```python
from build123d import *

# Parameters (mm, degrees)
F0_R     = 14.097
F0_R_2   = 14.1605
F0_R_3   = 14.224
F0_R_4   = 14.2875
F0_W     = 6.604
F0_H     = 13.208
F0_R_5   = 14.351
F0_H_2   = 12.954
F0_R_6   = 14.4145
F0_R_7   = 14.478
F1_DEPTH = 6.604


with BuildPart() as f1:
    # F0 (on Top) → F1 (new body)
    with BuildSketch(Plane.XY):
        with BuildLine():
            ThreePointArc((25.4, 123.19), (24.284077, 125.884077), (21.59, 127))
            Line((21.59, 127), (6.239323, 127))
            Line((6.239323, 127), (6.239323, 133.604))
            Line((6.239323, 133.604), (-6.460677, 133.604))
            Line((-6.460677, 133.604), (-6.460677, 127))
            Line((-6.460677, 127), (-21.59, 127))
            ThreePointArc((-21.59, 127), (-24.284077, 125.884077), (-25.4, 123.19))
            Line((-25.4, 123.19), (-25.4, -123.19))
            ThreePointArc((-25.4, -123.19), (-24.284077, -125.884077), (-21.59, -127))
            Line((-21.59, -127), (21.59, -127))
            ThreePointArc((21.59, -127), (24.284077, -125.884077), (25.4, -123.19))
            Line((25.4, -123.19), (25.4, 123.19))
        make_face()
        with Locations((0, -105.552882)):
            Circle(F0_R, mode=Mode.SUBTRACT)
        with Locations((0, -72.061613)):
            Circle(F0_R_2, mode=Mode.SUBTRACT)
        with Locations((0, -37.917089)):
            Circle(F0_R_3, mode=Mode.SUBTRACT)
        Circle(F0_R_4, mode=Mode.SUBTRACT)
        with Locations((20.013824, -19.935825)):
            Rectangle(F0_W, F0_H, mode=Mode.SUBTRACT)
        with Locations((0, 36.432702)):
            Circle(F0_R_5, mode=Mode.SUBTRACT)
        with Locations((18.755223, 17.765409)):
            Rectangle(F0_W, F0_H_2, mode=Mode.SUBTRACT)
        with Locations((0, 71.722105)):
            Circle(F0_R_6, mode=Mode.SUBTRACT)
        with Locations((0, 107.080773)):
            Circle(F0_R_7, mode=Mode.SUBTRACT)
    extrude(amount=F1_DEPTH)


solid = f1.part
```
Could you check a few things on this model? Use its own coordinates, in mm. A direction names the side the tool comes from. Coordinates: 2 decimals unless noted, no trailing zeros. Order: outer loops, then holes, each group sorted by start corner. A loop starts at its lowest first (then second) coordinate and runs counter-clockwise, first axis right, second up. Notation, with made-up numbers: M -22.5,65 L -17.5,65 A32 cw -17.5,100 Z; hole C 8,-19 d6. An arc over 180 degrees is marked long. Use a Markdown table: item, result. Add a question column.
Q1. We'd pull the mould along X, two halves only. Please class faces 5 (the flat face through (-17, 5, 6.604)), 6 (the cylindrical face through (-3.139, 92.947, 3.256)), 7 (the flat face through (6.239, 130, 3)): pulls with the +X half, pulls with the -X half, needs draft (parallel to the pull), parting line crosses it, or undercut.
Q2. I want a section at B-B on y = 0. List the corners of the cut face in (x, z) for me, then the cut area to 3 significant figures.
Q3. If I drill on L1, parallel to Y at x = 21, z = 1.25; L2, parallel to X at y = 105, z = 3.5; L3, parallel to Y at x = 16, z = 0.5, over which ranges is the centre line in solid material (lowest first)?
Q4. I want a section at A-A on x = 0. Give the number of separate pieces and of enclosed holes in the cut face, then the cut area to 3 significant figures.
Q5. I'm going to push flat-ended pins straight in: pin 1 (3.5 mm diameter, centred on x = -11, z = 3, fed in from +Y); pin 2 (6 mm diameter, centred on x = -13, y = -80, fed in from -Z). Where does each tip first touch, or does it pass through?
Q6. I want a section at D-D on y = 103. List the corners of the cut face in (x, z) for me, then the cut area to 3 significant figures.
Q7. Which directions (+Z, -Z, +X, -X, +Y, -Y) give clear straight access to the entire face, cutting with the end or side of a thin tool? Please do faces 1 (the flat face through (19, 11.288, 3)), 2 (the flat face through (-25.4, 2, 3)), 3 (the flat face through (14, 127, 3)), 4 (the flat face through (-6.461, 130, 3)).
Checked values:
| question | item | result |
|---|---|---|
| 1 | face 5 | needs draft |
| 1 | face 6 | undercut |
| 1 | face 7 | pulls with the +X half |
| 2 | outline | M -25.4,0 L -14.29,0 L -14.29,6.6 L -25.4,6.6 Z; M 14.29,0 L 25.4,0 L 25.4,6.6 L 14.29,6.6 Z |
| 2 | area | 147 mm² |
| 3 | L1 | -127 to -26.54, -13.33 to 11.29, 24.24 to 127 |
| 3 | L2 | -25.4 to -14.33, 14.33 to 25.4 |
| 3 | L3 | -127 to 11.29, 24.24 to 127 |
| 4 | separate pieces | 8 |
| 4 | enclosed holes | 0 |
| 4 | area | 400 mm² |
| 5 | pin 1 | y = 127 |
| 5 | pin 2 | z = 0 |
| 6 | outline | M -25.4,0 L -13.89,0 L -13.89,6.6 L -25.4,6.6 Z; M 13.89,0 L 25.4,0 L 25.4,6.6 L 13.89,6.6 Z |
| 6 | area | 152 mm² |
| 7 | face 1 | +Z, -Z |
| 7 | face 2 | +Z, -Z, -X, +Y, -Y |
| 7 | face 3 | +Z, -Z, +X, +Y |
| 7 | face 4 | +Z, -Z, -X, +Y |
